Part model, mm, in its own coordinate system. Face numbers are marked on the shaded views. Round coordinates to 2 decimals unless told otherwise and drop trailing zeros. Loops run counter-clockwise (first coordinate to the right, second up) from the corner with the lowest first, then second, coordinate; pieces in that order, holes last. Notation, with made-up numbers: (65.25, 64) -> (83.25, 64) arc R11 cw to (83.25, 72) -> close; hole circle Ø8 at (23.5, 89.25). An arc over 180 degrees is marked (long way). Use a Markdown table: item, result. Add a question column.
Item 1: Cut at D-D, the plane y = 5. State how many separate pieces and enclosed holes the cut face has, plus the area to 3 significant figures.
Item 2: Probe line 1 (Z direction, x = -12, y = 1.25); line 2 (Y direction, x = -40.5, z = -30); line 3 (Z direction, x = -55, y = -0.25). List the from-to ranges inside material, lowest first. Write a range as [from, to].
Item 3: Flat gauge pins, fed straight in: pin 1 (0.5 mm diameter, centred on x = -5, y = 0.5, fed in from -Z); pin 2 (1.5 mm diameter, centred on x = -52, z = -4.5, fed in from +Y); pin 3 (1.1 mm diameter, centred on x = -55.5, z = -32, fed in from +Y). Where does each tip first touch, or does it go through?
Item 4: Cut at B-B, the plane x = -45. List the corners of the cut face in (y, z), plus the area to 3 significant figures.
Item 5: Cut at A-A, the plane y = -1. List the corners of the cut face in (x, z), plus the area to 3 significant figures.
Item 6: Cut at C-C, the plane z = -26. List the corners of the cut face in (x, y), plus the area to 3 significant figures.
Item 7: Two-plate mould, pull along X, no slides. Class the marked faces 1 and 2: pulls with the +X half, pulls with the -X half, needs draft (parallel to the pull), parting line crosses it, or undercut.
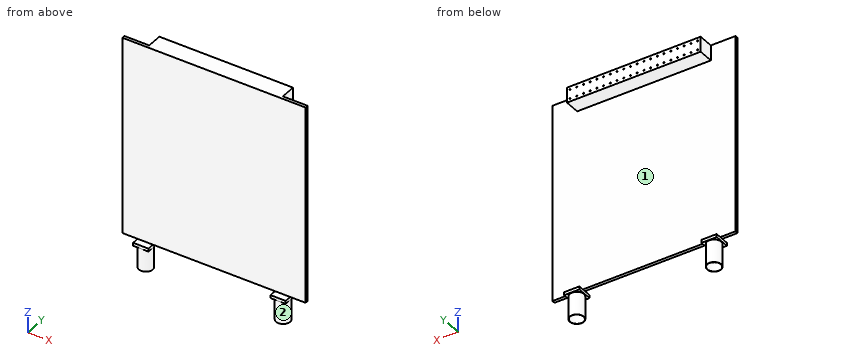
```python
from build123d import *

# Parameters (mm, degrees)
SKETCH_1_W                  = 60
SKETCH_1_H                  = 65
EXTRUDE_1_DEPTH             = 1
SKETCH_7_W                  = 43.8
SKETCH_7_H                  = 5
EXTRUDE_3_DEPTH             = 5
SKETCH_8_R                  = 0.2
CUT_EXTRUDE_2_DEPTH         = 5
PATTERN_LINEAR_1_COUNT      = 20
PATTERN_LINEAR_1_PITCH      = 2.2
PATTERN_LINEAR_1_COUNT_DIR2 = 2
PATTERN_LINEAR_1_PITCH_DIR2 = 3
SKETCH_9_W                  = 5
SKETCH_9_H                  = 5
EXTRUDE_4_DEPTH             = 1
SKETCH_10_R                 = 2.3
EXTRUDE_5_DEPTH             = 7.5
SKETCH_11_R                 = 2.2
CUT_EXTRUDE_3_DEPTH         = 7.5
PATTERN_LINEAR_2_COUNT      = 2
PATTERN_LINEAR_2_PITCH      = 45


with BuildPart() as part:
    # 草图1 → 凸台-拉伸1 (new body)
    with BuildSketch(Plane(origin=(0, 0, 0), x_dir=(1, 0, 0), z_dir=(0, 1, 0))):
        with Locations((-31.923076923, -0.769230769)):
            Rectangle(SKETCH_1_W, SKETCH_1_H)
    extrude(amount=EXTRUDE_1_DEPTH)

    # 草图7 → 凸台-拉伸3 (add)
    with BuildSketch(Plane(origin=(0, 1, 0), x_dir=(1, 0, 0), z_dir=(0, 1, 0))):
        with Locations((-31.923076923, -30.769230769)):
            Rectangle(SKETCH_7_W, SKETCH_7_H)
    extrude(amount=EXTRUDE_3_DEPTH)

    # 草图8 → 切除-拉伸2 (cut)
    with BuildSketch(Plane(origin=(0, 6, 0), x_dir=(1, 0, 0), z_dir=(0, 1, 0))):
        with Locations(Location((-52.823076923, -29.269230769, 0), (0, 0, 270))):
            Circle(SKETCH_8_R)
    cut_extrude_2 = extrude(amount=-CUT_EXTRUDE_2_DEPTH, mode=Mode.SUBTRACT)

    # 阵列(线性)1: Cut-Extrude 2 20 × 2
    with Locations(*[(i * PATTERN_LINEAR_1_PITCH, 0, j * PATTERN_LINEAR_1_PITCH_DIR2) for i in range(PATTERN_LINEAR_1_COUNT) for j in range(PATTERN_LINEAR_1_COUNT_DIR2) if (i, j) != (0, 0)]):
        add(cut_extrude_2, mode=Mode.SUBTRACT)

    # 草图9 → 凸台-拉伸4 (add)
    with BuildSketch(Plane(origin=(0, 0, -31.730769231), x_dir=(-1, 0, 0), z_dir=(0, 0, -1))):
        with Locations((9.423076923, 0.25)):
            Rectangle(SKETCH_9_W, SKETCH_9_H)
    extrude_4 = extrude(amount=EXTRUDE_4_DEPTH)

    # 草图10 → 凸台-拉伸5 (add)
    with BuildSketch(Plane(origin=(0, 0, -32.730769231), x_dir=(-1, 0, 0), z_dir=(0, 0, -1))):
        with Locations((9.423076923, 0.25)):
            Circle(SKETCH_10_R)
    extrude_5 = extrude(amount=EXTRUDE_5_DEPTH)

    # 草图11 → 切除-拉伸3 (cut)
    with BuildSketch(Plane(origin=(0, 0, -40.230769231), x_dir=(-1, 0, 0), z_dir=(0, 0, -1))):
        with Locations((9.423076923, 0.25)):
            Circle(SKETCH_11_R)
    cut_extrude_3 = extrude(amount=-CUT_EXTRUDE_3_DEPTH, mode=Mode.SUBTRACT)

    # 阵列(线性)2: 凸台-拉伸4, 凸台-拉伸5, 切除-拉伸3 ×2
    with Locations(*[(-i * PATTERN_LINEAR_2_PITCH, 0, 0) for i in range(1, PATTERN_LINEAR_2_COUNT)]):
        add(extrude_4)
        add(extrude_5)
        add(cut_extrude_3, mode=Mode.SUBTRACT)


solid = part.part
```
A:
| question | item | result |
|---|---|---|
| 1 | separate pieces | 1 |
| 1 | enclosed holes | 40 |
| 1 | area | 214 mm^2 |
| 2 | line 1 | z = [28.27, 33.27] |
| 2 | line 2 | y = [0, 1] |
| 2 | line 3 | z = [-32.73, -31.73] |
| 3 | pin 1 | stops at z = -31.73 |
| 3 | pin 2 | stops at y = 1 |
| 3 | pin 3 | stops at y = 2.75 |
| 4 | outline | (0, -31.73) -> (1, -31.73) -> (1, 28.27) -> (6, 28.27) -> (6, 33.27) -> (0, 33.27) -> close |
| 4 | area | 90.0 mm^2 |
| 5 | outline | (-56.92, -32.73) -> (-56.35, -32.73) -> (-56.35, -40.23) -> (-56.23, -40.23) -> (-56.23, -32.73) -> (-52.61, -32.73) -> (-52.61, -40.23) -> (-52.49, -40.23) -> (-52.49, -32.73) -> (-51.92, -32.73) -> (-51.92, -31.73) -> (-56.92, -31.73) -> close; (-11.92, -32.73) -> (-11.35, -32.73) -> (-11.35, -40.23) -> (-11.23, -40.23) -> (-11.23, -32.73) -> (-7.61, -32.73) -> (-7.61, -40.23) -> (-7.49, -40.23) -> (-7.49, -32.73) -> (-6.92, -32.73) -> (-6.92, -31.73) -> (-11.92, -31.73) -> close |
| 5 | area | 13.6 mm^2 |
| 6 | outline | (-61.92, 0) -> (-1.92, 0) -> (-1.92, 1) -> (-61.92, 1) -> close |
| 6 | area | 60.0 mm^2 |
| 7 | face 1 | needs draft |
| 7 | face 2 | undercut |
